Part print with two shaded views. Sizes in mm from the minimum x, y, z corner. A direction names the side the tool comes from. Round coordinates to 2 decimals unless told otherwise and drop trailing zeros. Order: outer loops, then holes, each group sorted by start corner. A loop starts at its lowest first (then second) coordinate and runs counter-clockwise, first axis right, second up. Notation, with made-up numbers: (37, 50) - (76, 50) arc R18 ccw to (76, 75) - close; hole circle Ø4 at (81, 25). An arc over 180 degrees is marked (long way). Use one line per item in the form item = value.
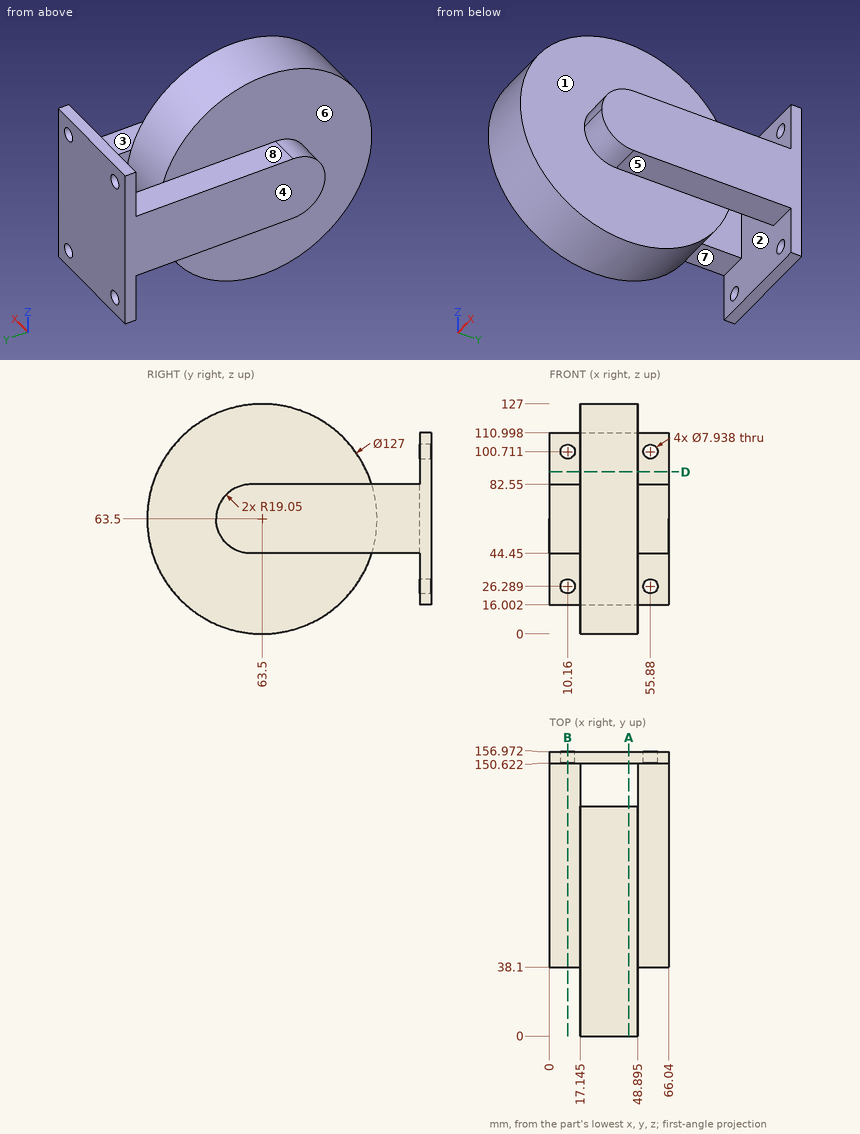
(1) Probe probe 1 along Z at (x, y) = (10, 155) (1 decimal); probe 2 along X at (y, z) = (128.5, 66.5) (1 decimal); probe 3 along Z at (x, y) = (55, 154). List the from-to ranges inside material, lowest first. Write a range as [from, to].
Report:
probe_1 = [16, 22.3], [30.3, 96.7], [104.7, 111]
probe_2 = [0, 17.1], [48.9, 66]
probe_3 = [16, 22.42], [30.16, 96.84], [104.58, 111]
(2) Slice it at A-A on x = 44. Give the cut face in (y, z), then the cut area to 3 significant figures.
Report:
outline = circle Ø127 at (63.5, 63.5); (150.62, 16) - (156.97, 16) - (156.97, 111) - (150.62, 111) - close
area = 13,300 mm2
(3) Pull direction X, two halves, no side cores. Call the marked faces 1, 2, 3 and 4: released by +X, released by -X, zero draft, split by the parting line, or undercut.
Report:
face_1 = released by +X
face_2 = undercut
face_3 = zero draft
face_4 = released by -X
(4) Slice it at D-D on z = 89.5. Give the cut face in (x, y) (1 decimal).
Report:
outline = (0, 150.6) - (66, 150.6) - (66, 157) - (0, 157) - close; (17.1, 5.6) - (48.9, 5.6) - (48.9, 121.4) - (17.1, 121.4) - close
(5) Tool access for the marked faces 5, 6, 7 and 8: list every direction of +Z, -Z, +X, -X, +Y, -Y with a clear straight run to the whole face (end or side of a thin tool).
Report:
face_5 = -Z, +X, -Y
face_6 = -X, -Y
face_7 = -Z, -X, -Y
face_8 = +Z, -X, -Y
(6) Pin check, flat tips, straight feed: pin 1 (5 mm diameter, centred on x = 57, y = 91, fed in from -Z); pin 2 (3 mm diameter, centred on x = 38.5, y = 153.5, fed in from +Z); pin 3 (12.5 mm diameter, centred on x = 55.88, z = 100.711, fed in from +Y); pin 4 (7 mm diameter, centred on x = 41, y = 153.5, fed in from -Z). Stop position of each tip, or through.
Report:
pin_1 = 44.45
pin_2 = 111
pin_3 = 156.97
pin_4 = 16
(7) Slice it at B-B on x = 10.16. Count the separate pieces of the cut face and the enclosed holes in it, then the cut area to 3 significant figures.
Report:
separate_pieces = 3
enclosed_holes = 0
area = 4,630 mm2
